Source: CAD feature listing. Evaluate the final solid. Frame: model axes, mm. Face numbers are marked on the shaded views. A direction names the side the tool comes from. Round coordinates to 2 decimals unless told otherwise and drop trailing zeros. Loops run counter-clockwise (first coordinate to the right, second up) from the corner with the lowest first, then second, coordinate; pieces in that order, holes last.
(1) Section A-A, the plane x = 16.5. Return the cut outline in (y, z).
(2) First-contact query: pin 1 Ø3 at (y, z) = (7.5, -2.5) entering from -X; pin 2 Ø2 at (y, z) = (0.5, -4.5) entering from -X; pin 3 Ø6 at (y, z) = (-27.5, -12.5) entering from -X. Flat tips, straight axial feed; report the tip coordinate or a pass-through.
(3) Section B-B, the plane y = -29. Return the cut outline in (x, z).
(4) Mould query, pull axis X, two halves, no side actions, for the marked faces 4, 5, 6 and 7. Classes: pulls with the +X half, pulls with the -X half, needs draft (parallel to the pull), parting line crosses it, or undercut.
(5) Set-up query: the marked faces 1, 2 and 3. Return all of +Z, -Z, +X, -X, +Y, -Y with unobstructed straight access to the full face (end or side cutting, diameter ignored); none if empty.
(6) Section D-D, the plane y = 1. Count the separate pieces of the cut face and the enclosed holes in it, plus the area to 3 significant figures.
(7) Material intervals for probe 1 along X at (y, z) = (17.75, -19.7); probe 2 along X at (y, z) = (20.55, -5); probe 3 along Z at (x, y) = (-7.5, 14.35), sorted ascending.
(8) Section C-C, the plane x = -17.5. Return the cut outline in (y, z).
```python
from build123d import *

# Parameters (mm, degrees)
PAD006_DEPTH            = 10
FILLET001_R             = 3
PAD013_DEPTH            = 10
SKETCH022_R             = 4.09
SKETCH022_W             = 2.5
SKETCH022_H             = 5.73
SKETCH022_W_2           = 5.73
SKETCH022_H_2           = 2.5
POCKET013_DEPTH         = 10.001
POCKET013_DEPTH_BACK    = 0.001
SKETCH023_R             = 1.5
POCKET014_DEPTH         = 7.5
SKETCH024_R             = 1.5
PAD019_DEPTH            = 8
SKETCH043_R             = 2.85
POCKET026_DEPTH         = 57.001
SKETCH047_R             = 1.5
POCKET029_DEPTH         = 5
SKETCH048_R             = 1.5
POCKET030_DEPTH         = 5
BODY005_ROLL_ANGLE      = -90
BODY005_PLACEMENT_ANGLE = 180


with BuildPart() as part:
    # Sketch006 → Pad006 (new body)
    with BuildSketch(Plane.XZ):
        with BuildLine():
            Line((18.25, 57), (12.25, 57))
            Line((12.25, 57), (0, 0))
            Line((0, 0), (0, -2.5))
            Line((0, -2.5), (50, -2.5))
            Line((50, -2.5), (50, 0))
            Line((50, 0), (37.75, 57))
            Line((37.75, 57), (31.75, 57))
            Line((31.25, 41.54951), (31.75, 57))
            ThreePointArc((31.75, 39), (31.623821, 40.299038), (31.25, 41.54951))
            Line((31.749951, 8.5), (31.75, 39))
            ThreePointArc((18.249951, 8.5), (24.999951, 7), (31.749951, 8.5))
            Line((18.25, 39), (18.249951, 8.5))
            ThreePointArc((18.75, 41.54951), (18.376179, 40.299038), (18.25, 39))
            Line((18.75, 41.54951), (18.25, 57))
        make_face()
    extrude(amount=-PAD006_DEPTH)

    # Fillet001
    fillet001_edges = [part.edges().sort_by_distance(p)[0] for p in [
        (31.749976, 10, 23.75),
        (18.249976, 10, 23.75),
        (18.376179, 10, 40.299038),
        (31.623821, 10, 40.299038),
    ]]
    fillet(fillet001_edges, radius=FILLET001_R)

    # Sketch021 → Pad013 (join)
    with BuildSketch(Plane.XZ):
        with BuildLine():
            ThreePointArc((15.25, 25.166146), (-4.5, 18.5), (15.25, 11.833854))
            Line((15.25, 25.166146), (15.25, 11.833854))
        make_face()
        with BuildLine():
            ThreePointArc((34.75, 11.833854), (54.5, 18.5), (34.75, 25.166146))
            Line((34.75, 25.166146), (34.75, 11.833854))
        make_face()
    extrude(amount=-PAD013_DEPTH)

    # Sketch022 → Pocket013 (cut, two sides)
    with BuildSketch(Plane.XZ) as pocket013_sk:
        with Locations((43.5, 18.5)):
            Circle(SKETCH022_R)
        with Locations((6.5, 18.5)):
            Circle(SKETCH022_R)
        with Locations((-0.78181, 18.5)):
            Rectangle(SKETCH022_W, SKETCH022_H)
        with Locations((50.78181, 18.5)):
            Rectangle(SKETCH022_W, SKETCH022_H)
        with Locations((32.5, 2.25)):
            Rectangle(SKETCH022_W_2, SKETCH022_H_2)
        with Locations((17.5, 2.25)):
            Rectangle(SKETCH022_W_2, SKETCH022_H_2)
    extrude(amount=-POCKET013_DEPTH, mode=Mode.SUBTRACT)
    extrude(pocket013_sk.sketch, amount=POCKET013_DEPTH_BACK, mode=Mode.SUBTRACT)

    # Sketch023 → Pocket014 (cut, symmetric)
    with BuildSketch(Plane.XY):
        with Locations((17.5, 5)):
            Circle(SKETCH023_R)
        with Locations((32.5, 5)):
            Circle(SKETCH023_R)
    extrude(amount=POCKET014_DEPTH, both=True, mode=Mode.SUBTRACT)

    # Sketch024 → Pad019 (join)
    with BuildSketch(Plane.XY.offset(-2.5)):
        Polygon((57, 0), (57, 24), (37, 24), (37, 0), (50, 0), align=None)
        with Locations((52.4, 19.7)):
            Circle(SKETCH024_R, mode=Mode.SUBTRACT)
        Polygon((-7, 24), (-7, 0), (0, 0), (13, 0), (13, 24), align=None)
        with Locations((-2.4, 19.7)):
            Circle(SKETCH024_R, mode=Mode.SUBTRACT)
    extrude(amount=PAD019_DEPTH)

    # Sketch043 → Pocket026 (cut, through all)
    with BuildSketch(Plane.XY):
        with Locations((-2.4, 19.7)):
            Circle(SKETCH043_R)
        with Locations((52.4, 19.7)):
            Circle(SKETCH043_R)
    extrude(amount=POCKET026_DEPTH, mode=Mode.SUBTRACT)

    # Sketch047 (on DatumPlane) → Pocket029 (cut, symmetric)
    with BuildSketch(Plane(origin=(52.03181, 0, 0), x_dir=(0, 0, -1), z_dir=(-1, 0, 0))):
        with Locations((-18.5, -5)):
            Circle(SKETCH047_R)
    extrude(amount=POCKET029_DEPTH, both=True, mode=Mode.SUBTRACT)

    # Sketch048 (on DatumPlane) → Pocket030 (cut, symmetric)
    with BuildSketch(Plane(origin=(-2.03181, 0, 0), x_dir=(0, 0, 1), z_dir=(1, 0, 0))):
        with Locations((18.5, -5)):
            Circle(SKETCH048_R)
    extrude(amount=POCKET030_DEPTH, both=True, mode=Mode.SUBTRACT)


with BuildPart() as part_1:
    # Body005 roll: moved
    add(part.part.rotate(Axis((0, 0, 0), (1, 0, 0)), BODY005_ROLL_ANGLE))


with BuildPart() as part_2:
    # Body005 placement: moved
    add(part_1.part.moved(Location((25, 19.5, 0))).rotate(Axis((25, 19.5, 0), (0, 0, 1)), BODY005_PLACEMENT_ANGLE))


solid = part_2.part
```
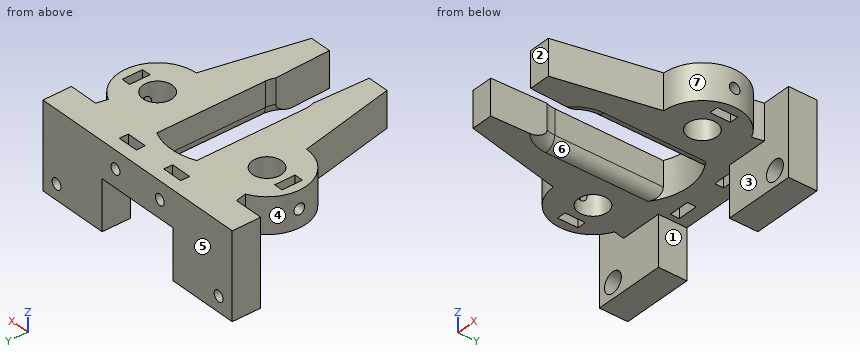
Output values:
1. outline: (-20.05, -10) - (-2.57, -10) - (-2.57, 0) - (-20.05, 0) - close; (4.57, -10) - (14, -10) - (14, -24) - (22, -24) - (22, 0) - (4.57, 0) - close
2. pin 1: stops at x = -28.3
2. pin 2: stops at x = -29.5
2. pin 3: stops at x = -15.26
3. outline: (-14.58, -10) - (-6.47, -10) - (-6.47, 0) - (-14.58, 0) - close; (6.47, -10) - (14.58, -10) - (14.58, 0) - (6.47, 0) - close
4. face 4: pulls with the -X half
4. face 5: needs draft
4. face 6: undercut
4. face 7: pulls with the +X half
5. face 1: -Z, +Y, -Y
5. face 2: +Z, -Z, +X, -X, -Y
5. face 3: -Z, +X
6. separate pieces: 10
6. enclosed holes: 0
6. area: 211 mm2
7. probe 1: x = -32 to -30.25, -24.55 to -12, 12 to 24.55, 30.25 to 32
7. probe 2: x = -32 to -9, -6 to 6, 9 to 32
7. probe 3: z = -10 to -6.5, -3.5 to 0
8. outline: (-15.4, -10) - (-2.97, -10) - (-2.97, 0) - (-15.4, 0) - close; (4.97, -10) - (14, -10) - (14, -24) - (22, -24) - (22, 0) - (4.97, 0) - close
